Geometry check sheet. Reference: the model listing, model coordinates, mm. Face numbers are marked on the shaded views. A direction names the side the tool comes from. Coordinates: 2 decimals unless noted, no trailing zeros. Write each question's results on one line, items separated by ' | '. Start each with the question number.
(1) Mould release check, pull along X, two halves, no side actions. Record for the marked faces 3, 4 and 5: pulls with the +X half, pulls with the -X half, needs draft (parallel to the pull), parting line crosses it, or undercut.
(2) Material ranges on probe 1 along X at (y, z) = (-17, -32); probe 2 along Z at (x, y) = (-42.5, 29.25); probe 3 along Z at (x, y) = (21.25, 26.75), recorded low to high.
(3) Go/stop test with flat-tipped pins: pin 1 Ø10 at (x, z) = (31.5, 19) entering from +Y; pin 2 Ø6 at (y, z) = (0, -35) entering from -X; pin 3 Ø1 at (x, z) = (21.5, -7.5) entering from +Y; pin 4 Ø2.5 at (x, z) = (-21.25, 36.81) entering from +Y. Record where each tip stops, or that it passes through.
(4) Access from +Z, -Z, +X, -X, +Y, -Y to the whole of each face (thin tool, end or side, straight path). Record for the marked faces 1 and 2.
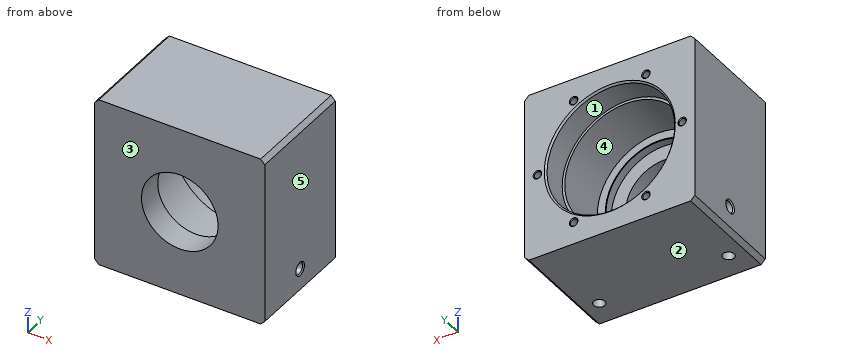
Autodesk Inventor part; units mm, degrees
ref_plane "YZ Plane" through (0, 0, 0) normal (1, 0, 0) x (0, 1, 0)
ref_plane "XZ Plane" through (0, 0, 0) normal (0, 1, 0) x (-1, 0, 0)
ref_plane "XY Plane" through (0, 0, 0) normal (0, 0, 1) x (1, 0, 0)
sketch "Skizze1" plane through (0, 0, 0) normal (0, 1, 0) x (-1, 0, 0)
  line L0 (0, -50) -> (-50, -50)
  line L1 (-50, -50) -> (-50, 50)
  line L2 (-50, 50) -> (0, 50)
  line L3 (0, -50) -> (50, -50)
  line L4 (50, -50) -> (50, 50)
  line L5 (50, 50) -> (0, 50)
  line L6 (-122.5, 0) -> (122.5, 0) construction
  line L7 (0, -77.2) -> (0, 113.2) construction
  dimension "d1" = 100
  dimension "d3" = 100
extrude "Grundkoerper" add sketch "Skizze1" along normal mid plane 65
sketch "Skizze2" plane through (0, -32.5, 0) normal (0, -1, 0) x (1, 0, 0)
  line L0 (-50, -50) -> (50, -50)
  line L1 (50, 50) -> (-50, 50)
  point P0 (0, 0)
  point P1 (0, 0)
  point P2 (-87.5, 0)
  point P3 (87.5, 0)
  dimension "d8" = 0
sketch "Skizze3" plane through (0, 0, 0) normal (1, 0, 0) x (0, 1, 0)
  line L0 (49, 0) -> (-49, 0) construction
  line L1 (-32.5, 50) -> (-32.5, -50) construction
  line L2 (32.5, -50) -> (32.5, 50) construction
  line L3 (17.5, 36) -> (-12.5, 36)
  line L4 (-12.5, 36) -> (-12.5, 31)
  line L5 (-17.5, 22.5) -> (-32.5, 22.5)
  line L6 (-32.5, -50) -> (-32.5, 50)
  line L7 (-32.5, 22.5) -> (-32.5, 0)
  line L8 (-32.5, 0) -> (32.5, 0)
  line L9 (32.5, 0) -> (32.5, 37.5)
  line L10 (-12.5, 31) -> (-17.5, 31)
  line L11 (-17.5, 31) -> (-17.5, 22.5)
  line L12 (17.5, 36) -> (17.5, 37.5)
  line L13 (17.5, 37.5) -> (32.5, 37.5)
  point P0 (0, 0)
  dimension "d9" = 45
  dimension "d10" = 72
  dimension "d11" = 45
  dimension "d33" = 5
  dimension "d34" = 62
  dimension "d160" = 75
  dimension "d161" = 30
revolve "Lagersitz" cut sketch "Skizze3" angle 360 about axis through (0, -32.5, 0) along (0, -1, 0)
sketch "Skizze_Lagersitz" plane through (0, 0, 0) normal (1, 0, 0) x (0, 1, 0)
  line L0 (-12.5, 36) -> (17.5, 36)
  line L1 (-12.5, -36) -> (-12.5, 36)
  line L2 (-17.5, 31) -> (-12.5, 31)
  line L3 (-17.5, -31) -> (-17.5, 31)
  line L4 (-32.5, 22.5) -> (-17.5, 22.5)
  line L5 (-32.5, -22.5) -> (-17.5, -22.5)
  line L6 (-17.5, -31) -> (-12.5, -31)
  line L7 (-12.5, -36) -> (17.5, -36)
  line L8 (32.5, 50) -> (32.5, -50)
  line L9 (30, -50) -> (30, 0)
  line L10 (-32.5, -22.5) -> (-32.5, 22.5)
  line L11 (-32.5, 50) -> (-32.5, -50)
  line L12 (-32.5, -50) -> (-32.5, 50)
  line L13 (-12.5, -36) -> (-12.5, 36)
  line L14 (17.5, -37.5) -> (17.5, 37.5)
  line L15 (17.5, 37.5) -> (32.5, 37.5)
  point P0 (0, 0)
  point P1 (30, 86)
  point P2 (30, 14)
  point P3 (-30, 32)
  point P4 (-30, 68)
  point P5 (32.5, 36)
  point P6 (32.5, -36)
sketch "Skizze5" plane through (0, 32.5, 0) normal (0, 1, 0) x (1, 0, 0)
  line L0 (0, 77.2) -> (0, -113.2) construction
  circle A0 centre (0, 0) radius 42.5 construction
  line L1 (122.5, 0) -> (-122.5, 0) construction
  point P0 (42.5, 0)
  point P1 (21.25, 36.8061)
  point P2 (-21.25, 36.8061)
  point P3 (-42.5, 0)
  point P4 (-21.25, -36.8061)
  point P5 (21.25, -36.8061)
  dimension "d167" = 85
  dimension "d170" = 360
hole "M5x10_Deckel" at (42.5, 32.5, 0) at (21.25, 32.5, -36.8061) at (-21.25, 32.5, -36.8061) at (-42.5, 32.5, 0) at (-21.25, 32.5, 36.8061) at (21.25, 32.5, 36.8061) direction (0, -1, 0) diameter 4.134 depth 14.2 tip angle 118 countersink diameter 5 countersink angle 90
sketch "Skizze9" plane through (50, -32.5, -50) normal (1, 0, 0) x (0, 0, -1)
  line L0 (-50, 81.5) -> (-50, -16.5) construction
  line L1 (0, 65) -> (0, 0) construction
  line L2 (-100, 65) -> (0, 65) construction
  line L3 (0, 0) -> (-100, 0) construction
  line L4 (-163.2, 32.5) -> (27.2, 32.5) construction
  point P0 (-50, 32.5)
  point P1 (-15, 32.5)
  dimension "d94" = 50
  dimension "d95" = 15
hole "M8x16_Seite" at (50, 0, -35) direction (-1, 0, 0) diameter 6.647 depth 22.2 tip angle 118 countersink diameter 8 countersink angle 90
mirror "M8x16_Seite_Spiegel" about plane through (0, 0, 0) normal (1, 0, 0) of "M8x16_Seite"
sketch "Skizze16" plane through (50, 32.5, -50) normal (0, 0, -1) x (-1, 0, 0)
  line L0 (50, -78) -> (50, 13) construction
  line L1 (100, -65) -> (0, -65) construction
  line L2 (100, 0) -> (100, -65)
  point P0 (50, -32.5)
  point P1 (88, -50)
  point P2 (12, -50)
  dimension "d181" = 76
  dimension "d182" = 15
  dimension "d183" = 12
hole "M8x16_Boden" at (-38, -17.5, -50) at (38, -17.5, -50) direction (0, 0, 1) diameter 6.647 depth 22.2 tip angle 118
chamfer "Fase_Lagersitz" distance 0.25 angle 45 1 edges at (0, -12.5, -31)
chamfer "Fase_Deckel" distance 1 angle 45 1 edges at (0, 32.5, -37.5)
chamfer "Fase_Allgemein" distance 2.5 angle 45 4 edges at (50, 0, 50) (-50, 0, 50) (50, 0, -50) (-50, 0, -50)
properties part number "200-10-ROCKER-BEARING-01" material "Aluminium 6061"
Outcome:
1) face 3: needs draft | face 4: undercut | face 5: pulls with the +X half
2) probe 1: x = -50 to -41.29, -34.71 to 34.71, 41.29 to 50 | probe 2: z = -50 to -2.07, 2.07 to 50 | probe 3: z = -50 to -38.87, -34.74 to -30.9, 30.9 to 34.74, 38.87 to 50
3) pin 1: stops at y = 32.5 | pin 2: stops at x = -27.61 | pin 3: stops at y = -17.5 | pin 4: stops at y = 17.81
4) face 1: +Y | face 2: -Z, +X, -X, +Y, -Y
